from build123d import *

# Parameters (mm, degrees)
F1_DEPTH     = 5
F2_R         = 12.7
F3_T1_DEPTH  = 5
F3_T3_DEPTH  = 5
F3_T5_DEPTH  = 5
F3_T7_DEPTH  = 5
F3_T9_DEPTH  = 14.2270901057
F3_T11_DEPTH = 18.0454684025
F4_R         = 1.27
F5_R         = 9.652
F6_T1_DEPTH  = 24.5237287856
F6_T3_DEPTH  = 20.8349691576
F6_T5_DEPTH  = 25.4326352389


# Not quite as in the source:
# - a fillet or chamfer that OpenCascade refuses, or shapes differently, is made with other operations: its cross-section is extruded or revolved along the edge and cut away or added


with BuildPart() as f1:
    # F0 (on Top) → F1 (new body)
    with BuildSketch(Plane.XY):
        Polygon((3.3509032068, 2.0938767152), (4.2717468935, 6.0824889279), (5.2645709983, 10.3828825854), (-0.7663700033, 9.1009665025), (-1.7591941081, 4.800572845), (-2.0938767152, 3.3509032068), (0, 0), align=None)
        with BuildLine():
            ThreePointArc((19.0271173058, -10.7843702882), (13.5579507926, -11.3055566189), (8.4773948837, -9.2147746604))
            Line((8.4773948837, -9.2147746604), (3, -9.3617991862))
            Line((3, -9.3617991862), (-3, -9.5228515064))
            Line((-3, -9.5228515064), (-24.13, -10.0900240941))
            Line((-24.13, -10.0900240941), (-24.13, -6.5340240941))
            Line((-24.13, -6.5340240941), (-24.13, -4.0344355705))
            Line((-24.13, -4.0344355705), (-25.33, -4.0344355705))
            Line((-25.33, -4.0344355705), (-25.33, -13.3233871439))
            Line((-25.33, -13.3233871439), (-20.25, -13.1870295128))
            Line((-20.25, -13.1870295128), (-10.09, -12.9143142505))
            Line((-10.09, -12.9143142505), (15.568160115, -12.2255965474))
            ThreePointArc((15.568160115, -12.2255965474), (27.3847553183, 1.4414639293), (12.6972400213, 11.962745157))
            Line((12.6972400213, 11.962745157), (5.2645709983, 10.3828825854))
            Line((5.2645709983, 10.3828825854), (4.2717468935, 6.0824889279))
            Line((4.2717468935, 6.0824889279), (5.7705051289, 6.4010598252))
            ThreePointArc((5.7705051289, 6.4010598252), (10.9582466373, 10.5977114577), (17.6052347625, 11.1826009729))
            ThreePointArc((17.6052347625, 11.1826009729), (26.6461306142, 0.7382983213), (19.0271173058, -10.7843702882))
        make_face()
        Polygon((-24.13, -4.0344355705), (-24.13, -6.5340240941), (-22.86, -6.7579593596), align=None)
        Polygon((-3, -9.5228515064), (3, -9.3617991862), (3, 1.222), (0, -1.778), (-3, 1.222), align=None)
        Polygon((-1.7591941081, 4.800572845), (-0.7663700033, 9.1009665025), (-10.09, 7.1191677681), (-20.25, 4.9595931015), (-20.6003244103, 4.8851293494), (-23.2697767574, 2.48154366), (-25.4, 3.8649268089), (-25.4, 2.5949268089), (-23.9501636865, 0.0837366513), align=None)
        with BuildLine():
            Line((5.7705051289, 6.4010598252), (17.6052347625, 11.1826009729))
            ThreePointArc((17.6052347625, 11.1826009729), (10.9582466373, 10.5977114577), (5.7705051289, 6.4010598252))
        make_face()
        with BuildLine():
            Line((19.0271173058, -10.7843702882), (8.4773948837, -9.2147746604))
            ThreePointArc((8.4773948837, -9.2147746604), (13.5579507926, -11.3055566189), (19.0271173058, -10.7843702882))
        make_face()
        with BuildLine():
            Line((-20.25, 4.9595931015), (-10.09, 7.1191677681))
            Line((-10.09, 7.1191677681), (-10.09, 9.660082633))
            ThreePointArc((-10.09, 9.660082633), (-15.1017802383, 6.9821995552), (-20.25, 9.3873673708))
            Line((-20.25, 9.3873673708), (-20.25, 4.9595931015))
        make_face()
        with BuildLine():
            Line((-10.09, -17.0008412983), (-10.09, -12.9143142505))
            Line((-10.09, -12.9143142505), (-20.25, -13.1870295128))
            Line((-20.25, -13.1870295128), (-20.25, -17.2735565605))
            ThreePointArc((-20.25, -17.2735565605), (-15.2382197617, -14.5956734827), (-10.09, -17.0008412983))
        make_face()
    extrude(amount=F1_DEPTH)

    # F2
    f2_edges = [f1.edges().sort_by_distance(p)[0] for p in [
        (5.770505, 6.40106, 2.5),
        (8.477395, -9.214775, 2.5),
    ]]
    fillet(f2_edges, radius=F2_R)

    # F3: fillet of radius 2.54 on 8 edges, made by hand

    # F3_s2 → F3_t1 (join)
    with BuildSketch(Plane.XY):
        with BuildLine():
            ThreePointArc((5.6695141413, 6.421250807), (4.5433342643, 5.7258928643), (3.9198768127, 4.5583721621))
            Line((3.9198768127, 4.5583721621), (3.6723868163, 4.6155097299))
            Line((3.6723868163, 4.6155097299), (4.024256897, 6.1396264957))
            Line((4.024256897, 6.1396264957), (4.218937324, 6.3309384185))
            ThreePointArc((4.218937324, 6.3309384185), (4.6308698651, 6.4184973831), (5.5969878777, 6.6646762393))
            Line((5.5969878777, 6.6646762393), (5.6695141413, 6.421250807))
        make_face()
    extrude(amount=F3_T1_DEPTH)

    # F3_s4 → F3_t3 (join)
    with BuildSketch(Plane.XY):
        with BuildLine():
            ThreePointArc((-2.0938767152, 3.3509032068), (-3.2128527644, 4.1204303422), (-4.5683542412, 4.2034674259))
            Line((-4.5683542412, 4.2034674259), (-1.7591941081, 4.800572845))
            Line((-1.7591941081, 4.800572845), (-2.0938767152, 3.3509032068))
        make_face()
    extrude(amount=F3_T3_DEPTH)

    # F3_s6 → F3_t5 (join)
    with BuildSketch(Plane.XY):
        with BuildLine():
            ThreePointArc((5.6081542675, -9.2917909701), (3.7682087933, -8.5726933957), (3, -6.7527055057))
            Line((3, -6.7527055057), (3, -9.3617991862))
            Line((3, -9.3617991862), (5.6081542675, -9.2917909701))
        make_face()
    extrude(amount=F3_T5_DEPTH)

    # F3_s8 → F3_t7 (join)
    with BuildSketch(Plane.XY):
        with BuildLine():
            ThreePointArc((-3, -7.050115457), (-3.72001211, -8.8219066637), (-5.4718457325, -9.5892009215))
            Line((-5.4718457325, -9.5892009215), (-3, -9.5228515064))
            Line((-3, -9.5228515064), (-3, -7.050115457))
        make_face()
    extrude(amount=F3_T7_DEPTH)

    # F3_s10 → F3_t9 (cut)
    with BuildSketch(Plane.XY.offset(-4.6135450528)):
        with BuildLine():
            ThreePointArc((-24.872872697, 1.6819155382), (-23.7062792448, 0.6315100757), (-22.1450724768, 0.4674206323))
            Line((-22.1450724768, 0.4674206323), (-23.9501636865, 0.0837366513))
            Line((-23.9501636865, 0.0837366513), (-24.872872697, 1.6819155382))
        make_face()
    extrude(amount=F3_T9_DEPTH, mode=Mode.SUBTRACT)

    # F3_s12 → F3_t11 (cut)
    with BuildSketch(Plane.XY.offset(-6.5227342013)):
        with BuildLine():
            ThreePointArc((-22.7218457325, -13.2533789278), (-24.5617912067, -12.5342813534), (-25.33, -10.7142934634))
            Line((-25.33, -10.7142934634), (-25.33, -13.3233871439))
            Line((-25.33, -13.3233871439), (-22.7218457325, -13.2533789278))
        make_face()
    extrude(amount=F3_T11_DEPTH, mode=Mode.SUBTRACT)

    # F4
    f4_edges = [f1.edges().sort_by_distance(p)[0] for p in [
        (-24.13, -10.090024, 2.5),
    ]]
    fillet(f4_edges, radius=F4_R)

    # F5
    f5_edges = [f1.edges().sort_by_distance(p)[0] for p in [
        (17.605235, 11.182601, 2.5),
        (19.027117, -10.78437, 2.5),
    ]]
    fillet(f5_edges, radius=F5_R)

    # F6: fillet of radius 2.032 on 4 edges, made by hand

    # F6_s2 → F6_t1 (cut)
    with BuildSketch(Plane.XY.offset(-9.7618643928)):
        with BuildLine():
            ThreePointArc((-20.25, 5.4826216137), (-19.3751275367, 7.152974829), (-17.5038584017, 7.3849953356))
            ThreePointArc((-17.5038584017, 7.3849953356), (-19.0133811971, 8.1990450487), (-20.25, 9.3873673708))
            Line((-20.25, 9.3873673708), (-20.25, 5.4826216137))
        make_face()
        with BuildLine():
            ThreePointArc((-12.8361415983, -14.9984692631), (-10.9648724633, -14.7664487565), (-10.09, -13.0960955412))
            Line((-10.09, -13.0960955412), (-10.09, -17.0008412983))
            ThreePointArc((-10.09, -17.0008412983), (-11.3266188029, -15.8125189761), (-12.8361415983, -14.9984692631))
        make_face()
    extrude(amount=F6_T1_DEPTH, mode=Mode.SUBTRACT)

    # F6_s4 → F6_t3 (cut)
    with BuildSketch(Plane.XY.offset(-7.9174845788)):
        with BuildLine():
            ThreePointArc((-12.5069745437, 7.613601755), (-11.2148663887, 7.7751542861), (-10.09, 7.1191677681))
            Line((-10.09, 7.1191677681), (-10.09, 9.660082633))
            ThreePointArc((-10.09, 9.660082633), (-11.1688571334, 8.4837438934), (-12.5069745437, 7.613601755))
        make_face()
    extrude(amount=F6_T3_DEPTH, mode=Mode.SUBTRACT)

    # F6_s6 → F6_t5 (cut)
    with BuildSketch(Plane.XY.offset(-10.2163176194)):
        with BuildLine():
            ThreePointArc((-20.25, -13.1870295128), (-19.3485712422, -14.8643401762), (-17.4543465947, -15.0589111198))
            ThreePointArc((-17.4543465947, -15.0589111198), (-19.0108515696, -15.9659266289), (-20.25, -17.2735565605))
            Line((-20.25, -17.2735565605), (-20.25, -13.1870295128))
        make_face()
    extrude(amount=F6_T5_DEPTH, mode=Mode.SUBTRACT)


solid = f1.part
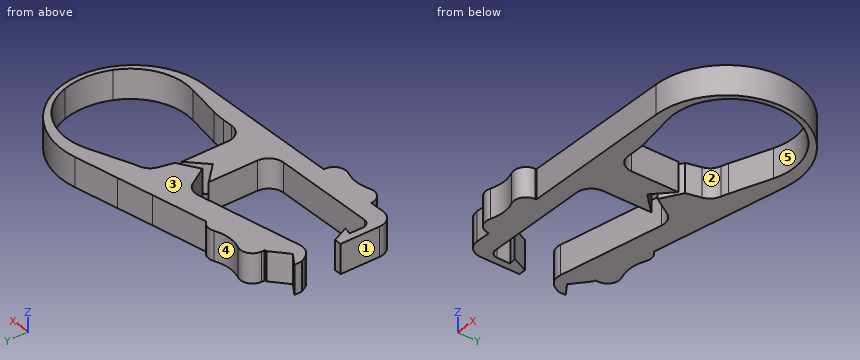
CAD build for the part. Positions are in the model's coordinates, mm. Face numbers are marked on the shaded views. A direction names the side the tool comes from. Round coordinates to 2 decimals unless told otherwise and drop trailing zeros. Order: outer loops, then holes, each group sorted by start corner. A loop starts at its lowest first (then second) coordinate and runs counter-clockwise, first axis right, second up. Notation, with made-up numbers: (40.5, 46.5) - (55.5, 46.5) arc R30 ccw to (55.5, 70.5) - close; hole circle Ø11 at (9.25, -35.75). An arc over 180 degrees is marked (long way). Return JSON: item names as keys, results as strings.
(1) Cut at A-A (x = 21). Give the cut face in (y, z), then the cut area to 3 significant figures.
Answer key:
{"outline": "(-10.79, 0) - (-9.43, 0) - (-9.43, 5) - (-10.79, 5) - close; (9.26, 0) - (10.79, 0) - (10.79, 5) - (9.26, 5) - close", "area": "14.4 mm^2"}
(2) Cut at B-B (y = -2.5). Give the cut face in (x, z), then the cut area to 3 significant figures.
Answer key:
{"outline": "(-3, 0) - (3, 0) - (3, 5) - (-3, 5) - close; (26.39, 0) - (27.21, 0) - (27.21, 5) - (26.39, 5) - close", "area": "34.1 mm^2"}
(3) Tool access for the marked faces 4 and 5: list every direction of +Z, -Z, +X, -X, +Y, -Y with a clear straight run to the whole face (end or side of a thin tool).
Answer key:
{"face 4": "+Z, -Z, +Y", "face 5": "+Z, -Z"}
(4) Pull direction X, two halves, no side cores. Call the marked faces 1, 2 and 3: +X half, -X half, draft (parallel to the pull), parting line (faces both ways), or undercut.
Answer key:
{"face 1": "-X half", "face 2": "undercut", "face 3": "draft"}
(5) Pin check, flat tips, straight feed: pin 1 Ø2.5 at (y, z) = (-4.5, 3) entering from +X; pin 2 Ø1.1 at (y, z) = (-7.5, 3.5) entering from +X; pin 3 Ø3 at (x, z) = (3.5, 2) entering from +Y. Stop position of each tip, or through.
Answer key:
{"pin 1": "stops at x = 27.03", "pin 2": "stops at x = 25.3", "pin 3": "stops at y = 10.33"}
(6) Wall check: probe 1 along X at (y, z) = (-6, 1.5); probe 2 along Y at (x, z) = (-19, 2.9); probe 3 along X at (y, z) = (-2, 2.8). Give the ranges that are in metal, low to high. Write a range as from..to.
Answer key:
{"probe 1": "x = -25.33..-23.21, -3..3, 24.94..25.9", "probe 2": "y = -15.05..-9.95, 1.14..7.36", "probe 3": "x = -3..3, 26.49..27.31"}
